```python
from build123d import *

# Parameters (mm, degrees)
SKETCH009_R          = 10
PAD007_DEPTH         = 8
SKETCH010_R          = 5
PAD008_DEPTH         = 19
SKETCH011_R          = 2
POCKET001_DEPTH      = 10.001
POCKET001_DEPTH_BACK = 10.001


with BuildPart() as part:
    # Sketch009 → Pad007 (new body)
    with BuildSketch(Plane.XY):
        Circle(SKETCH009_R)
    extrude(amount=-PAD007_DEPTH)

    # Sketch010 → Pad008 (join)
    with BuildSketch(Plane.XY):
        Circle(SKETCH010_R)
    extrude(amount=PAD008_DEPTH)

    # Sketch011 → Pocket001 (cut, two sides)
    with BuildSketch(Plane.YZ) as pocket001_sk:
        with Locations((0, 12)):
            Circle(SKETCH011_R)
    extrude(amount=-POCKET001_DEPTH, mode=Mode.SUBTRACT)
    extrude(pocket001_sk.sketch, amount=POCKET001_DEPTH_BACK, mode=Mode.SUBTRACT)


solid = part.part
```
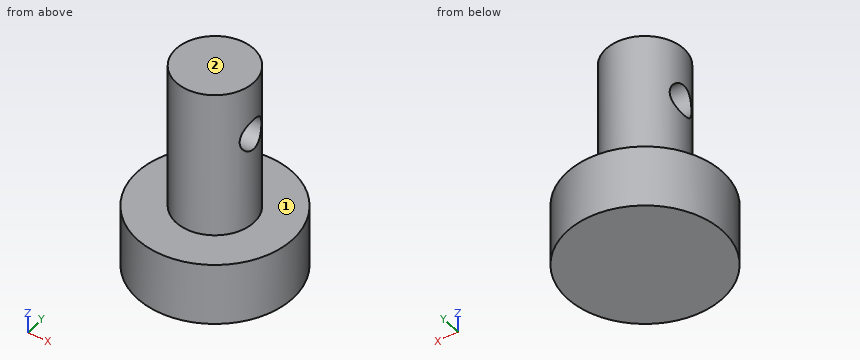
Input: part model. Units: mm. Frame: model coordinates. Face numbers are marked on the shaded views. A direction names the side the tool comes from. Coordinates: 2 decimals unless noted, no trailing zeros. Write each loop counter-clockwise with the first axis right and the second up, starting at its lowest first coordinate (ties: lowest second). Pieces come first, ordered by that corner, then holes.
1) Section C-C on z = 4.75. Output: boundary loops of the cut face in (x, y), and give its area (3 significant figures).
2) Pin query (flat end, axial travel): pin 1 Ø3.5 at (y, z) = (0, 12) entering from -X; pin 2 Ø5 at (y, z) = (-4, 7.5) entering from -X; pin 3 Ø4 at (y, z) = (-3, 10) entering from -X; pin 4 Ø6 at (y, z) = (4, -2.5) entering from -X. Return the tip coordinate at first contact, or that it passes through.
3) Section D-D on y = 6. Output: boundary loops of the cut face in (x, z), and give its area (3 significant figures).
4) Material intervals for line 1 along Z through (x, y) = (1.2, 0); line 2 along Z through (x, y) = (3.75, -7.5); line 3 along Y through (x, z) = (-2.7, 12), sorted ascending.
5) Section A-A on y = 0. Output: boundary loops of the cut face in (x, z), and give its area (3 significant figures).
6) Set-up query: the marked faces 1 and 2. Return all of +Z, -Z, +X, -X, +Y, -Y with unobstructed straight access to the full face (end or side cutting, diameter ignored); none if empty.
7) Section B-B on x = -0.75. Output: boundary loops of the cut face in (y, z), and give its area (3 significant figures).
Check result:
1. outline: circle Ø10 at (0, 0)
1. area: 78.5 mm2
2. pin 1: passes through
2. pin 2: stops at x = -4.77
2. pin 3: stops at x = -4.9
2. pin 4: stops at x = -9.95
3. outline: (-8, -8) - (8, -8) - (8, 0) - (-8, 0) - close
3. area: 128 mm2
4. line 1: z = -8 to 10, 14 to 19
4. line 2: z = -8 to 0
4. line 3: y = -4.21 to -2, 2 to 4.21
5. outline: (-10, -8) - (10, -8) - (10, 0) - (5, 0) - (5, 10) - (-5, 10) - (-5, 0) - (-10, 0) - close; (-5, 14) - (5, 14) - (5, 19) - (-5, 19) - close
5. area: 310 mm2
6. face 1: +Z
6. face 2: +Z, +X, -X, +Y, -Y
7. outline: (-9.97, -8) - (9.97, -8) - (9.97, 0) - (4.94, 0) - (4.94, 19) - (-4.94, 19) - (-4.94, 0) - (-9.97, 0) - close; hole circle Ø4 at (0, 12)
7. area: 335 mm2
